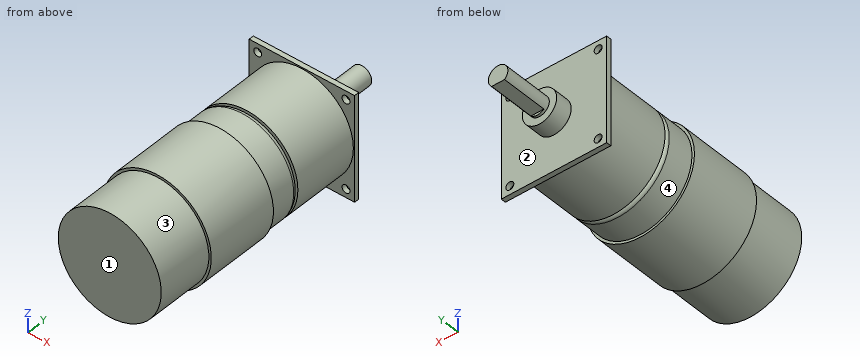
Autodesk Inventor part; units mm, degrees
ref_plane "Work Plane3" through (21, 33, 0) normal (1, 0, 0) x (0, 0, -1)
ref_plane "YZ Plane" through (0, 0, 0) normal (1, 0, 0) x (0, 1, 0)
ref_plane "XZ Plane" through (0, 0, 0) normal (0, 1, 0) x (-1, 0, 0)
sketch "Sketch1" plane through (0, 0, 0) normal (0, 1, 0) x (-1, 0, 0)
  circle A0 centre (0, 0) radius 21
  circle A1 centre (0, 0) radius 22
  dimension "d0" = 42
  dimension "d105" = 44
extrude "Extrusion1" add sketch "Sketch1" along normal mid plane 66 contours A0
fillet "Fillet1" radius 2 1 edges at (21, 33, 0)
sketch "Sketch2" plane through (0, 33, 0) normal (0, 1, 0) x (1, 0, 0)
  circle A0 centre (0, 0) radius 21
  dimension "d4" = 42
extrude "Extrusion2" add sketch "Sketch2" along normal blind 28.8
sketch "Sketch14" plane through (0, 61.8, 0) normal (0, 1, 0) x (1, 0, 0)
  line L0 (-21.5, 21.5) -> (21.5, 21.5)
  line L1 (21.5, 21.5) -> (21.5, -21.5)
  line L2 (21.5, -21.5) -> (-21.5, -21.5)
  line L3 (-21.5, -21.5) -> (-21.5, 21.5)
  line L4 (-21.5, 21.5) -> (21.5, -21.5) construction
  line L5 (21.5, 21.5) -> (-21.5, -21.5) construction
  point P0 (0, 0)
  dimension "d81" = 43
  dimension "d82" = 43
extrude "Extrusion13" add sketch "Sketch14" against normal blind 2
sketch "Sketch15" plane through (0, 61.8, 0) normal (0, 1, 0) x (1, 0, 0)
  point P0 (0, 0)
  point P1 (-18, 18)
  point P2 (18, 18)
  point P3 (18, -18)
  point P4 (-18, -18)
  dimension "d85" = 36
  dimension "d86" = 36
  dimension "d87" = 18
  dimension "d88" = 18
hole "Hole2" at (-18, 61.8, -18) at (18, 61.8, -18) at (18, 61.8, 18) at (-18, 61.8, 18) direction (0, -1, 0) diameter 3.242 end through all
sketch "Sketch16" plane through (0, 61.8, 0) normal (0, 1, 0) x (1, 0, 0)
  point P0 (0, 0)
sketch "Sketch17" plane through (0, 61.8, 0) normal (0, 1, 0) x (1, 0, 0)
  circle A0 centre (0, 0) radius 7
  dimension "d96" = 14
extrude "Extrusion14" add sketch "Sketch17" along normal blind 7
sketch "Sketch18" plane through (0, 68.8, 0) normal (0, 1, 0) x (1, 0, 0)
  circle A0 centre (0, 0) radius 4
  dimension "d99" = 8
extrude "Extrusion15" add sketch "Sketch18" along normal blind 20
sketch "Sketch19" plane through (0, 88.8, 0) normal (0, 1, 0) x (1, 0, 0)
  circle A0 centre (0, 0) radius 4
  line L0 (-2.6458, 3) -> (2.6458, 3)
  dimension "d102" = 3
extrude "Extrusion16" cut sketch "Sketch19" against normal blind 19 contours L0 A0 picked at (-0.6179, 3.1815)
extrude "Extrusion17" add sketch "Sketch1" along normal blind 20 and the other way blind 10
ref_plane "Work Plane3" through (21, 33, 0) normal (1, 0, 0) x (0, 0, -1)
sketch "Sketch20" plane through (21, 33, 0) normal (1, 0, 0) x (0, 0, -1)
  line L0 (20.5, 25.8) -> (20.5, 2.0287) construction
  line L1 (20.5, 2.0287) -> (-20.5, 2.0287) construction
  line L2 (-20.5, 2.0287) -> (-20.5, 25.8) construction
  line L3 (-20.5, 25.8) -> (20.5, 25.8) construction
  line L4 (21.5, 28.8) -> (21.5, 26.8)
  line L5 (-21.5, 28.8) -> (-21.5, 26.8)
  line L6 (21.5, 26.8) -> (-21.5, 26.8)
  point P0 (0, -33)
  dimension "d123" = 1
  dimension "d124" = 1
  dimension "d125" = 1
decal "Decal2"
properties part number "HCMUTE-CDT23-MOTOR_DC24V-100RPM-XD42GA775"
Verification items for the finished model (mm, model axes). Face numbers are marked on the shaded views. A direction names the side the tool comes from. Round coordinates to 2 decimals unless told otherwise and drop trailing zeros. Write each loop counter-clockwise with the first axis right and the second up, starting at its lowest first coordinate (ties: lowest second). Pieces come first, ordered by that corner, then holes. Notation, with made-up numbers: (72, 72) - (106, 72) arc R23 cw to (106, 100) - close; hole circle Ø1 at (53.25, 60.5). An arc over 180 degrees is marked (long way). Answer as a JSON object with one key per item and string values. Group by question number.
Q1. Section check C-C, the plane y = 65.5. Enter the section's corners in (x, z).
Q2. Go/stop test with flat-tipped pins: pin 1 Ø1 at (y, z) = (31, -17) entering from +X; pin 2 Ø13 at (x, z) = (-7, 8.5) entering from +Y; pin 3 Ø1.6 at (y, z) = (60.5, 2) entering from -X. Record where each tip stops, or that it passes through.
Q3. Section check D-D, the plane x = 18. Give the number of separate pieces and of enclosed holes in the cut face, plus the area to 3 significant figures.
Q4. Thickness scan on line 1 (X direction, y = 61, z = 18); line 2 (Y direction, x = 11, z = -4). Record the ranges inside material, lowest first.
Q5. Tool access check on the marked faces 1, 2, 3 and 4. Record the directions out of +Z, -Z, +X, -X, +Y, -Y that give a thin tool (end or side, any length) a straight path to the whole face; none if there is none.
Found:
{
 "1": {"outline": "circle Ø14 at (0, 0)"},
 "2": {"pin 1": "stops at x = 12.99", "pin 2": "stops at y = 68.8", "pin 3": "stops at x = -21.5"},
 "3": {"separate pieces": "3", "enclosed holes": "0", "area": "2,190 mm^2"},
 "4": {"line 1": "x = -21.5 to -19.62, -16.38 to 16.38, 19.62 to 21.5", "line 2": "y = -33 to 61.8"},
 "5": {"face 1": "+Z, -Z, +X, -X, -Y", "face 2": "+Y", "face 3": "-Y", "face 4": "none"}
}
